Autodesk Inventor part; units mm, degrees
ref_plane "YZ Plane" through (0, 0, 0) normal (1, 0, 0) x (0, 1, 0)
ref_plane "XZ Plane" through (0, 0, 0) normal (0, 1, 0) x (-1, 0, 0)
ref_plane "XY Plane" through (0, 0, 0) normal (0, 0, 1) x (1, 0, 0)
sketch "Sketch1" plane through (0, 0, 0) normal (1, 0, 0) x (0, 1, 0)
  line L0 (0, 0) -> (30, 0)
  line L1 (30, 0) -> (30, -30)
  line L2 (30, -30) -> (0, -30)
  line L3 (0, -30) -> (0, 0)
  line L4 (0, -8.4131) -> (10, -3.75)
  line L5 (10, -3.75) -> (10, -26.25)
  line L6 (10, -26.25) -> (0, -21.5869)
  point P0 (10, -15)
  point P1 (0, -15)
  dimension "d0" = 30
  dimension "d1" = 30
  dimension "d2" = 10
  dimension "d3" = 22.5
  dimension "d4" = 65
  dimension "d5" = 65
extrude "Extrusion1" add sketch "Sketch1" along normal blind 30 contours L0 L1 L2 L3 L6 L5 L4
sketch "Sketch2" plane through (30, 0, 0) normal (1, 0, 0) x (0, 0, -1)
  line L0 (0, 30) -> (0, 0)
  line L1 (21.5869, 0) -> (30, 0)
  line L2 (0, 30) -> (30, 30)
  line L3 (30, 30) -> (30, 0)
  line L4 (30, 0) -> (0, 0)
  line L5 (0, 0) -> (0, 30)
  point P0 (21.5869, 0)
extrude "Extrusion2" add sketch "Sketch2" along normal blind 2.5
sketch "Sketch3" plane through (0, 0, 0) normal (-1, 0, 0) x (0, 0, 1)
  line L0 (-30, 0) -> (-30, 30)
  line L1 (0, 30) -> (0, 0)
  line L2 (-30, 30) -> (0, 30)
  line L3 (0, 30) -> (0, 25)
  line L4 (0, 25) -> (-30, 25)
  line L5 (-30, 25) -> (-30, 30)
  point P0 (0, 30)
  dimension "d10" = 5
extrude "Extrusion3" add sketch "Sketch3" along normal blind 5
sketch "Sketch4" plane through (32.5, 30, 0) normal (0, 1, 0) x (1, 0, 0)
  line L0 (-32.5, 0) -> (-37.5, 0)
  line L1 (-32.5, 0) -> (-32.5, 30) construction
  circle A0 centre (-35, 15) radius 1.5
  dimension "d13" = 3
extrude "Extrusion4" cut sketch "Sketch4" against normal through all
sketch "Sketch5" plane through (32.5, 30, 0) normal (0, 1, 0) x (1, 0, 0)
  line L0 (-29.2486, 25.6211) -> (-4.7242, 25.6211)
  line L1 (-4.7242, 25.6211) -> (-4.7242, 4.3789)
  line L2 (-4.7242, 4.3789) -> (-29.2486, 4.3789)
  line L3 (-29.2486, 4.3789) -> (-29.2486, 25.6211)
  line L4 (0, 30) -> (0, 0)
  point P0 (-32.5, 0)
  point P1 (0, 15)
  point P2 (-4.7242, 15)
  point P3 (0, 15)
extrude "Extrusion5" cut sketch "Sketch5" against normal blind 19
sketch "Sketch6" plane through (32.5, 0, 0) normal (1, 0, 0) x (0, 0, -1)
  line L0 (25.6211, 11) -> (4.3789, 11)
  line L1 (10, 21) -> (20, 21)
  line L2 (20, 21) -> (20, 15)
  line L3 (20, 15) -> (10, 15)
  line L4 (10, 15) -> (10, 21)
  point P0 (0, 0)
  point P1 (15, 15)
  point P2 (15, 11)
  dimension "d18" = 10
  dimension "d19" = 6
  dimension "d20" = 4
extrude "Extrusion6" cut sketch "Sketch6" against normal up to next
properties part number "Top Sensor Mount"
CAD build for the part. Positions are in the model's coordinates, mm. A direction names the side the tool comes from. Coordinates: 2 decimals unless noted, no trailing zeros. Order: outer loops, then holes, each group sorted by start corner. A loop starts at its lowest first (then second) coordinate and runs counter-clockwise, first axis right, second up. Notation, with made-up numbers: (75, 4) - (99, 4) arc R19 cw to (99, 22) - close; hole circle Ø7 at (12.5, -15). An arc over 180 degrees is marked (long way). Use a Markdown table: item, result. Add a question column.
(1) Pull direction Y, two halves, no side cores. Call faces 4 (the face through (30, 18, -20)), 5 (the face through (14, 15, -30)), 6 (the face through (16, 0, -22)): +Y half, -Y half, draft (parallel to the pull), parting line (faces both ways), or undercut.
(2) Saw through at C-C (y = 13.5). Give the cut face in (x, z), then the cut area to 3 significant figures.
(3) Saw through at D-D (x = 17.5). Give the cut face in (y, z), then the cut area to 3 significant figures.
(4) Saw through at B-B (z = -15). Give the cut face in (x, y), then the cut area to 3 significant figures.
(5) Which spindle directions (+Z, -Z, +X, -X, +Y, -Y) get a long thin tool onto all of the face, cutting with end or side? Do faces 1 (the face through (0, 15, -15)), 2 (the face through (14.79, 4.93, -6.114)), 3 (the face through (3.251, 21, -15)). Say none if no direction does.
(6) Drill centre lines: line 1 along Z through (x, y) = (3.5, 21.5); line 2 along Z through (x, y) = (-2.5, 28.3); line 3 along X through (y, z) = (24.5, -5). Where is each one in solid material? Low to high. Write a range as [from, to].
(7) Flat gauge pins, fed straight in: pin 1 (10 mm diameter, centred on x = 10.5, z = -12.5, fed in from +Y); pin 2 (1 mm diameter, centred on x = 5, z = -19.5, fed in from -Y); pin 3 (2.5 mm diameter, centred on x = -2.5, z = -13.5, fed in from -Y). Where does each tip first touch, or does it go through?
(8) Saw through at A-A (x = -2.5). Give the cut face in (y, z), then the cut area to 3 significant figures.
Solved:
| question | item | result |
|---|---|---|
| 1 | face 4 | undercut |
| 1 | face 5 | draft |
| 1 | face 6 | -Y half |
| 2 | outline | (0, -30) - (32.5, -30) - (32.5, 0) - (0, 0) - close; hole (3.25, -25.62) - (27.78, -25.62) - (27.78, -4.38) - (3.25, -4.38) - close |
| 2 | area | 454 mm² |
| 3 | outline | (0, -30) - (30, -30) - (30, -25.62) - (11, -25.62) - (11, -4.38) - (30, -4.38) - (30, 0) - (0, 0) - (0, -8.41) - (10, -3.75) - (10, -26.25) - (0, -21.59) - close |
| 3 | area | 318 mm² |
| 4 | outline | (-5, 25) - (-4, 25) - (-4, 30) - (-5, 30) - close; (-1, 25) - (0, 25) - (0, 10) - (30, 10) - (30, 0) - (32.5, 0) - (32.5, 15) - (27.78, 15) - (27.78, 11) - (3.25, 11) - (3.25, 30) - (-1, 30) - close; (27.78, 21) - (32.5, 21) - (32.5, 30) - (27.78, 30) - close |
| 4 | area | 191 mm² |
| 5 | face 1 | +Z, -Z, -X, -Y |
| 5 | face 2 | -X |
| 5 | face 3 | +Y |
| 6 | line 1 | z = [-30, -25.62], [-4.38, 0] |
| 6 | line 2 | z = [-30, -16.5], [-13.5, 0] |
| 6 | line 3 | x = [0, 3.25], [27.78, 32.5] |
| 7 | pin 1 | stops at y = 11 |
| 7 | pin 2 | stops at y = 10 |
| 7 | pin 3 | stops at y = 25 |
| 8 | outline | (25, -30) - (30, -30) - (30, -16.5) - (25, -16.5) - close; (25, -13.5) - (30, -13.5) - (30, 0) - (25, 0) - close |
| 8 | area | 135 mm² |
